from build123d import *

# Parameters (mm, degrees)
SKETCH_1_W          = 16
SKETCH_1_H          = 16
SKETCH_1_R          = 1.5
SKETCH_1_R_2        = 0.8
SKETCH_1_R_3        = 0.4
EXTRUDE_1_DEPTH     = 3.6
CUT_EXTRUDE_START   = 3.6
SKETCH_1_3_R        = 2.3
CUT_EXTRUDE_1_DEPTH = 2.6
SKETCH_1_4_R        = 1
CUT_EXTRUDE_2_DEPTH = 2.6


with BuildPart() as part:
    # 草图1 → 凸台-拉伸1 (new body)
    with BuildSketch(Plane(origin=(0, 0, 0), x_dir=(1, 0, 0), z_dir=(0, 1, 0))):
        Rectangle(SKETCH_1_W, SKETCH_1_H)
        with Locations(Location((0, 0, 0), (0, 0, 270))):
            Circle(SKETCH_1_R, mode=Mode.SUBTRACT)
        with Locations(Location((-4, 4, 0), (0, 0, 270))):
            Circle(SKETCH_1_R_2, mode=Mode.SUBTRACT)
        with Locations(Location((4, 4, 0), (0, 0, 270))):
            Circle(SKETCH_1_R_2, mode=Mode.SUBTRACT)
        with Locations(Location((-4, -4, 0), (0, 0, 270))):
            Circle(SKETCH_1_R_2, mode=Mode.SUBTRACT)
        with Locations(Location((4, -4, 0), (0, 0, 270))):
            Circle(SKETCH_1_R_2, mode=Mode.SUBTRACT)
        with Locations(Location((-6, 6, 0), (0, 0, 270))):
            Circle(SKETCH_1_R_3, mode=Mode.SUBTRACT)
        with Locations(Location((6, 6, 0), (0, 0, 270))):
            Circle(SKETCH_1_R_3, mode=Mode.SUBTRACT)
        with Locations(Location((6, -6, 0), (0, 0, 270))):
            Circle(SKETCH_1_R_3, mode=Mode.SUBTRACT)
        with Locations(Location((-6, -6, 0), (0, 0, 270))):
            Circle(SKETCH_1_R_3, mode=Mode.SUBTRACT)
    extrude(amount=EXTRUDE_1_DEPTH)

    # 草图1<3> → 切除-拉伸1 (cut)
    with BuildSketch(Plane(origin=(0, 0, 0), x_dir=(1, 0, 0), z_dir=(0, 1, 0)).offset(CUT_EXTRUDE_START)):
        with Locations(Location((0, 0, 0), (0, 0, 270))):
            Circle(SKETCH_1_3_R)
    extrude(amount=-CUT_EXTRUDE_1_DEPTH, mode=Mode.SUBTRACT)

    # 草图1<4> → 切除-拉伸2 (cut)
    with BuildSketch(Plane(origin=(0, 0, 0), x_dir=(1, 0, 0), z_dir=(0, 1, 0))):
        with Locations(Location((-4, 4, 0), (0, 0, 270))):
            Circle(SKETCH_1_4_R)
        with Locations(Location((4, 4, 0), (0, 0, 270))):
            Circle(SKETCH_1_4_R)
        with Locations(Location((4, -4, 0), (0, 0, 270))):
            Circle(SKETCH_1_4_R)
        with Locations(Location((-4, -4, 0), (0, 0, 270))):
            Circle(SKETCH_1_4_R)
    extrude(amount=CUT_EXTRUDE_2_DEPTH, mode=Mode.SUBTRACT)


solid = part.part
Could you check a few things on this model? Use its own coordinates, in mm. A direction names the side the tool comes from. Give positions to 0.01 mm unless a question says otherwise; leave off trailing zeros. Order: outer loops, then holes, each group sorted by start corner. A loop starts at its lowest first (then second) coordinate and runs counter-clockwise, first axis right, second up.
1. Will these pins go through, and if not, where does the flat tip stop? P1, Ø1, axis at x = 4, z = -4, coming from the -Y side; P2, Ø1.8, axis at x = -4, z = -4, coming from the -Y side.
2. Suppose I cut it at D-D (x = 0). List the corners of the cut face in (y, z) for me.
3. I need wall thicknesses on L1, parallel to X at y = 2.1, z = -6; L2, parallel to X at y = 3.25, z = -4. Which ranges of each line are inside material? Lowest first, please.
4. Suppose I cut it at B-B (x = -6). List the corners of the cut face in (y, z) for me, plus the area to 3 significant figures.
5. Suppose I cut it at A-A (z = -4). List the corners of the cut face in (x, y) for me, plus the area to 3 significant figures.
6. For faces 1 (the cylindrical face through (-4, 1, -5)), 2 (the cylindrical face through (-4.49, 3.09, 3.37)), which set-ups out of +Z, -Z, +X, -X, +Y, -Y let a thin tool reach every point of the face, with its end or its side?
7. We'd pull the mould along X, two halves only. Please class faces 3 (the flat face through (-2, 3.6, -2)), 4 (the flat face through (-8, 2, 0)), 5 (the cylindrical face through (-4.49, 3.09, -4.63)): pulls with the +X half, pulls with the -X half, needs draft (parallel to the pull), parting line crosses it, or undercut.
8. Suppose I cut it at C-C (y = 2.1). Give the number of separate pieces and of enclosed holes in the cut face, plus the area to 3 significant figures.
Solved:
1. P1: passes through
1. P2: stops at y = 2.6
2. outline: (0, -8) - (3.6, -8) - (3.6, -2.3) - (1, -2.3) - (1, -1.5) - (0, -1.5) - close; (0, 1.5) - (1, 1.5) - (1, 2.3) - (3.6, 2.3) - (3.6, 8) - (0, 8) - close
3. L1: x = -8 to -6.4, -5.6 to 5.6, 6.4 to 8
3. L2: x = -8 to -4.8, -3.2 to 3.2, 4.8 to 8
4. outline: (0, -8) - (3.6, -8) - (3.6, -6.4) - (0, -6.4) - close; (0, -5.6) - (3.6, -5.6) - (3.6, 5.6) - (0, 5.6) - close; (0, 6.4) - (3.6, 6.4) - (3.6, 8) - (0, 8) - close
4. area: 51.8 mm2
5. outline: (-8, 0) - (-5, 0) - (-5, 2.6) - (-4.8, 2.6) - (-4.8, 3.6) - (-8, 3.6) - close; (-3.2, 2.6) - (-3, 2.6) - (-3, 0) - (3, 0) - (3, 2.6) - (3.2, 2.6) - (3.2, 3.6) - (-3.2, 3.6) - close; (4.8, 2.6) - (5, 2.6) - (5, 0) - (8, 0) - (8, 3.6) - (4.8, 3.6) - close
5. area: 44.0 mm2
6. face 1: -Y
6. face 2: +Y, -Y
7. face 3: needs draft
7. face 4: pulls with the -X half
7. face 5: undercut
8. separate pieces: 1
8. enclosed holes: 9
8. area: 225 mm2
